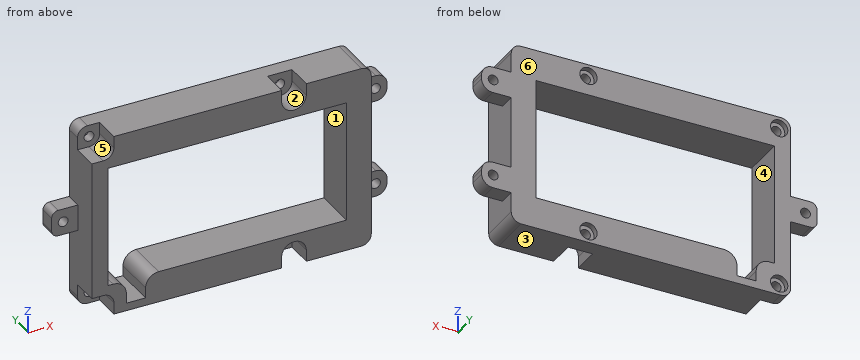
Autodesk Inventor part; units mm, degrees
ref_plane "YZ Plane" through (0, 0, 0) normal (1, 0, 0) x (0, 1, 0)
ref_plane "XZ Plane" through (0, 0, 0) normal (0, 1, 0) x (-1, 0, 0)
ref_plane "XY Plane" through (0, 0, 0) normal (0, 0, 1) x (1, 0, 0)
sketch "Sketch1" plane through (0, 0, 0) normal (0, 1, 0) x (-1, 0, 0)
  line L0 (-3, 0) -> (-82, 0)
  line L1 (-85, -3) -> (-85, -53)
  line L2 (-82, -56) -> (-3, -56)
  line L3 (0, -53) -> (0, -3)
  arc A0 (-3, -56) -> (0, -53) centre (-3, -53) ccw
  arc A1 (0, -3) -> (-3, 0) centre (-3, -3) ccw
  arc A2 (-82, 0) -> (-85, -3) centre (-82, -3) ccw
  arc A3 (-85, -53) -> (-82, -56) centre (-82, -53) ccw
  circle A4 centre (-3.5, -52.5) radius 1.5
  circle A5 centre (-3.5, -3.5) radius 1.5
  circle A6 centre (-61.5, -52.5) radius 1.5
  circle A7 centre (-61.5, -3.5) radius 1.5
  point P0 (0, 0)
  point P1 (-85, -56)
  point P2 (-85, 0)
  point P3 (0, -56)
  dimension "d0" = 85
  dimension "d1" = 56
  dimension "d2" = 3
  dimension "d9" = 3
  dimension "d10" = 3
  dimension "d15" = 3
  dimension "d16" = 3
  dimension "d140" = 58
  dimension "d141" = 58
  dimension "d142" = 49
  dimension "d143" = 3.5
extrude "Extrusion1" add sketch "Sketch1" along normal blind 13
sketch "Sketch12" plane through (0, 0, 0) normal (0, -1, 0) x (1, 0, 0)
  line L0 (5, -9.5) -> (77.5, -9.5)
  line L1 (77.5, -9.5) -> (77.5, -46.5)
  line L2 (5, -46.5) -> (5, -9.5)
  line L3 (82, -56) -> (3, -56)
  line L4 (85, -3) -> (85, -53)
  line L5 (3, 0) -> (82, 0)
  line L6 (0, -53) -> (0, -3)
  line L7 (16.35, -50.5) -> (16.35, -53.65)
  line L8 (16.35, -53.65) -> (10.5, -53.65)
  line L9 (10.5, -53.65) -> (10.5, -50.5)
  line L10 (77.5, -46.5) -> (20.35, -46.5)
  line L11 (6.5, -46.5) -> (5, -46.5)
  arc A0 (10.5, -50.5) -> (6.5, -46.5) centre (6.5, -50.5) ccw
  arc A1 (20.35, -46.5) -> (16.35, -50.5) centre (20.35, -50.5) ccw
  point P0 (0, 0)
  point P1 (10.5, -46.5)
  point P2 (16.35, -46.5)
  dimension "d153" = 7.5
  dimension "d154" = 9.5
  dimension "d155" = 5
  dimension "d157" = 10.5
  dimension "d158" = 2.35
  dimension "d159" = 5.85
  dimension "d160" = 4
extrude "Extrusion12" cut sketch "Sketch12" against normal up to next
sketch "Sketch14" plane through (0, 13, 0) normal (0, 1, 0) x (1, 0, 0)
  circle A0 centre (3.5, 3.5) radius 1.5
  circle A1 centre (3.5, 3.5) radius 2.625
  circle A2 centre (61.5, 3.5) radius 1.5
  circle A3 centre (61.5, 3.5) radius 2.625
  circle A4 centre (61.5, 52.5) radius 1.5
  circle A5 centre (61.5, 52.5) radius 2.625
  circle A6 centre (3.5, 52.5) radius 1.5
  circle A7 centre (3.5, 52.5) radius 2.625
  point P0 (0, 0)
  dimension "d161" = 5.25
  dimension "d162" = 5.25
  dimension "d163" = 5.25
  dimension "d164" = 5.25
extrude "Extrusion14" cut sketch "Sketch14" against normal blind 1.75 contours A0 | A1 | A2 | A3 | A4 | A5 | A6 | A7
sketch "Sketch15" plane through (0, 0, 0) normal (0, -1, 0) x (1, 0, 0)
  arc A0 (3.5, -6.75) -> (6.75, -3.5) centre (3.5, -3.5) ccw
  arc A1 (57.75, -3.5) -> (65.25, -3.5) centre (61.5, -3.5) ccw
  arc A2 (65.25, -52.5) -> (57.75, -52.5) centre (61.5, -52.5) ccw
  arc A3 (6.75, -52.5) -> (3.5, -49.25) centre (3.5, -52.5) ccw
  line L0 (57.75, -3.5) -> (57.75, 0)
  line L1 (3, 0) -> (82, 0)
  line L2 (65.25, -3.5) -> (65.25, 0)
  line L3 (65.25, -52.5) -> (65.25, -56)
  line L4 (82, -56) -> (3, -56)
  line L5 (57.75, -52.5) -> (57.75, -56)
  line L6 (6.75, -3.5) -> (6.75, 0)
  line L7 (3.5, -6.75) -> (0, -6.75)
  line L8 (0, -53) -> (0, -3)
  line L9 (3.5, -49.25) -> (0, -49.25)
  line L10 (6.75, -52.5) -> (6.75, -56)
  line L11 (65.25, 0) -> (57.75, 0)
  line L12 (65.25, -56) -> (57.75, -56)
  arc A4 (0, -53) -> (3, -56) centre (3, -53) ccw
  line L13 (6.75, -56) -> (3, -56)
  line L14 (0, -49.25) -> (0, -53)
  line L15 (0, -6.75) -> (0, -3)
  line L16 (3, 0) -> (6.75, 0)
  arc A5 (3, 0) -> (0, -3) centre (3, -3) ccw
  arc A6 (3, 0) -> (0, -3) centre (3, -3) ccw
  arc A7 (0, -53) -> (3, -56) centre (3, -53) ccw
  point P0 (0, 0)
  dimension "d167" = 6.5
  dimension "d168" = 6.5
  dimension "d169" = 7.5
  dimension "d170" = 7.5
extrude "Extrusion15" cut sketch "Sketch15" against normal blind 8.25
sketch "Sketch16" plane through (0, 13, 0) normal (0, 1, 0) x (1, 0, 0)
  line L0 (5, 9.5) -> (5, 46.5)
  line L1 (0, 49.25) -> (0, 6.75)
  line L2 (0, 32) -> (-6, 32)
  line L3 (-8, 30) -> (-8, 26)
  line L4 (-6, 24) -> (0, 24)
  line L5 (0, 24) -> (0, 32)
  circle A0 centre (-4.5, 28) radius 1.5
  arc A1 (-6, 32) -> (-8, 30) centre (-6, 30) ccw
  arc A2 (-8, 26) -> (-6, 24) centre (-6, 26) ccw
  line L6 (3, 0) -> (82, 0)
  line L7 (42.5, 0) -> (42.5, 9.5)
  line L8 (85, 39) -> (90.6651, 39)
  line L9 (94, 42.3349) -> (94, 43.6651)
  line L10 (90.6651, 47) -> (85, 47)
  line L11 (85, 47) -> (85, 39)
  circle A3 centre (90.5, 43) radius 1.5
  arc A4 (90.6651, 39) -> (94, 42.3349) centre (90.6651, 42.3349) ccw
  arc A5 (94, 43.6651) -> (90.6651, 47) centre (90.6651, 43.6651) ccw
  line L12 (85, 3) -> (85, 53)
  line L13 (82, 56) -> (3, 56)
  line L14 (85, 17) -> (85, 9)
  line L15 (90.6651, 17) -> (85, 17)
  line L16 (85, 9) -> (90.6651, 9)
  circle A6 centre (90.5, 13) radius 1.5
  arc A7 (94, 13.6651) -> (90.6651, 17) centre (90.6651, 13.6651) ccw
  line L17 (94, 12.3349) -> (94, 13.6651)
  arc A8 (90.6651, 9) -> (94, 12.3349) centre (90.6651, 12.3349) ccw
  point P0 (0, 0)
  point P1 (0, 28)
  point P2 (-8, 24)
  point P3 (-8, 32)
  point P4 (94, 47)
  point P5 (94, 39)
  point P6 (85, 28)
  point P7 (94, 17)
  point P8 (94, 9)
  point P9 (0, 24)
  dimension "d175" = 4
  dimension "d176" = 8
  dimension "d177" = 8
  dimension "d178" = 4
  dimension "d179" = 3.5
  dimension "d180" = 2
  dimension "d183" = 8
  dimension "d184" = 9
  dimension "d185" = 4
  dimension "d186" = 3.5
  dimension "d188" = 0
  dimension "d189" = 9
  dimension "d190" = 8
  dimension "d191" = 9
  dimension "d192" = 4
  dimension "d193" = 3.5
  dimension "d194" = 9
  dimension "d197" = 3
  dimension "d198" = 3
  dimension "d199" = 3
  dimension "d200" = 24
extrude "Extrusion16" add sketch "Sketch16" against normal blind 5
equation "\"d10\" = d9"
equation "\"d15\" = d9"
equation "\"d16\" = d9"
equation "\"d162\" = d161"
equation "\"d163\" = d161"
equation "\"d164\" = d161"
equation "\"d178\" = d175"
equation "\"d185\" = 0.5 * d183"
equation "\"d192\" = 0.5 * d190"
equation "\"d198\" = d197"
equation "\"d199\" = d197"
equation "\"d182\" = 0.5 * d183"
properties part number "Pi3BatteryBoard_Mockup"
Here's how the part is built. I have some questions about the finished solid (model axes, mm). Face numbers are marked on the shaded views. A direction names the side the tool comes from. Give positions to 0.01 mm unless a question says otherwise; leave off trailing zeros. Write each loop counter-clockwise with the first axis right and the second up, starting at its lowest first coordinate (ties: lowest second). Pieces come first, ordered by that corner, then holes.
(1) Imagine slicing it at D-D, the plane x = -4.5. Write out the boundary of the cut face in (y, z), and give its area (3 significant figures).
Output values:
outline: (8, -32) - (13, -32) - (13, -29.5) - (8, -29.5) - close; (8, -26.5) - (13, -26.5) - (13, -24) - (8, -24) - close
area: 25.0 mm2
(2) Imagine slicing it at B-B, the plane z = -37.5. Write out the boundary of the cut face in (x, y), and give its area (4 significant figures).
Output values:
outline: (0, 0) - (5, 0) - (5, 13) - (0, 13) - close; (77.5, 0) - (85, 0) - (85, 13) - (77.5, 13) - close
area: 162.5 mm2
(3) Imagine slicing it at A-A, the plane x = 61.5. Write out the boundary of the cut face in (y, z) (3 decimals), and give its area (3 significant figures).
Output values:
outline: (0, -48.75) - (8.25, -48.75) - (8.25, -51) - (11.25, -51) - (11.25, -49.875) - (13, -49.875) - (13, -46.5) - (0, -46.5) - close; (0, -9.5) - (13, -9.5) - (13, -6.125) - (11.25, -6.125) - (11.25, -5) - (8.25, -5) - (8.25, -7.25) - (0, -7.25) - close; (8.25, -56) - (13, -56) - (13, -55.125) - (11.25, -55.125) - (11.25, -54) - (8.25, -54) - close; (8.25, -2) - (11.25, -2) - (11.25, -0.875) - (13, -0.875) - (13, 0) - (8.25, 0) - close
area: 91.0 mm2
(4) Thinking about a two-plate mould opening in Z: for the marked faces 1, 2 and 3, which applies, pulls with the +Z half, pulls with the -Z half, needs draft (parallel to the pull), parting line crosses it, or undercut?
Output values:
face 1: undercut
face 2: pulls with the +Z half
face 3: pulls with the -Z half
(5) On a 3-axis mill with a long thin cutter (end or side, diameter ignored), from which of +Z, -Z, +X, -X, +Y, -Y can I reach the whole of each face in a straight line? I mean the marked faces 4, 5 and 6. Say none if no direction works.
Output values:
face 4: +Y, -Y
face 5: +Z, -X, -Y
face 6: +Z, -Z, +X, -X, +Y
(6) Will these pins go through, and if not, where does the flat tip stop? pin 1 (4 mm diameter, centred on y = 5, z = -54.5, fed in from -X); pin 2 (1.5 mm diameter, centred on x = 88, y = 10, fed in from +Z); pin 3 (5 mm diameter, centred on y = 3.5, z = -20.5, fed in from -X).
Output values:
pin 1: stops at x = 6.75
pin 2: stops at z = -9
pin 3: stops at x = 0
(7) If I drill on L1, parallel to X at y = 9.95, z = -13; L2, parallel to X at y = 12.1, z = -52.5 (3 decimals); L3, parallel to X at y = 9.7, z = -3.5, over which ranges is the centre line in solid material (lowest first)?
Output values:
L1: x = 0 to 5, 77.5 to 89, 92 to 94
L2: x = 0 to 0.875, 6.125 to 10.5, 16.35 to 58.875, 64.125 to 85
L3: x = 0 to 2, 5 to 60, 63 to 85
